Check sheet for the modelled part. Datum: model origin and axes. Units: mm. Coordinates: 2 decimals unless noted, no trailing zeros. Write each loop counter-clockwise with the first axis right and the second up, starting at its lowest first coordinate (ties: lowest second). Pieces come first, ordered by that corner, then holes. Notation, with made-up numbers: (-23.75, 63) -> (-0.75, 63) arc R7 ccw to (-0.75, 73) -> close; hole circle Ø9 at (14, 85.25). An arc over 180 degrees is marked (long way). One line per item, written item: value. Start each with the question number.
1) Draft check along Z on faces 1 (the cylindrical face through (-46.367, 225.4, -60.47)), 2 (the cylindrical face through (23.54, 225.4, 74.74)), 3 (the flat face through (66.1, 0, -38.4)). Enter one of: +Z half, -Z half, draft (parallel to the pull), parting line (faces both ways), or undercut.
2) Sectioned sample at C-C on y = 287.5. Enter the section's corners in (x, z).
3) Sectioned sample at A-A on z = 0. Enter the section's corners in (x, y).
4) Scan lines: line 1 along Z through (x, y) = (0, 292); line 2 along Y through (x, z) = (0, 76.7); line 3 along Z through (x, y) = (52, 426.5). Record each from-to range of solid material in increasing order. Write a range as [from, to].
5) Gauge pin test, flat ends, axial feed: P1, Ø5, axis at x = 19, y = 296, coming from the -Z side; P2, Ø6, axis at x = 62, y = 115, coming from the +Z side; P3, Ø5, axis at x = -47, y = 353.5, coming from the +Z side; P4, Ø2, axis at x = 0, y = 4.76, coming from the -Z side. Record the tip position at first contact, or that the pin passes through.
6) Sectioned sample at B-B on x = 53. Enter the section's corners in (y, z).
```python
from build123d import *

# Parameters (mm, degrees)
SKETCH1_R               = 78.359
SKETCH1_R_2             = 76.2
BOSS_EXTRUDE1_DEPTH     = 457.2
SKETCH2_R               = 1.750000056
CUT_EXTRUDE1_DEPTH      = 471.438206104
CIRPATTERN1_COUNT       = 6
CUT_EXTRUDE2_REACH      = 491.625
CUT_EXTRUDE2_END_RADIUS = 76.2
CIRPATTERN2_COUNT       = 3


with BuildPart() as part:
    # Sketch1 → Boss-Extrude1 (new body)
    with BuildSketch(Plane(origin=(0, 0, 0), x_dir=(1, 0, 0), z_dir=(0, 1, 0))):
        with Locations(Location((0, 0, 0), (0, 0, 270))):
            Circle(SKETCH1_R)
        with Locations(Location((0, 0, 0), (0, 0, 270))):
            Circle(SKETCH1_R_2, mode=Mode.SUBTRACT)
    extrude(amount=BOSS_EXTRUDE1_DEPTH)

    # Sketch2 → Cut-Extrude1 (cut, through all)
    with BuildSketch(Plane.XY):
        with Locations(Location((0, 4.7625, 0), (0, 0, 90))):
            Circle(SKETCH2_R)
    cut_extrude1 = extrude(amount=-CUT_EXTRUDE1_DEPTH, mode=Mode.SUBTRACT)

    # CirPattern1: Cut-Extrude1 ×6 about axis
    cirpattern1_axis = Axis((0, 457.2, 0), (0, -1, 0))
    for i in range(1, CIRPATTERN1_COUNT):
        add(cut_extrude1.rotate(cirpattern1_axis, i * 360 / CIRPATTERN1_COUNT), mode=Mode.SUBTRACT)

    # Cut-Extrude2: up to this cylinder (the profile starts outside it)
    cut_extrude2_end = Plane(origin=(0, 3.909431, 0), z_dir=(0, -1, 0)) * Cylinder(CUT_EXTRUDE2_END_RADIUS, 1136.65, mode=Mode.PRIVATE)
    # Sketch3 → Cut-Extrude2 (cut, up to the surface)
    with BuildSketch(Plane(origin=(0, 0, -78.359), x_dir=(-1, 0, 0), z_dir=(0, 0, -1)), mode=Mode.PRIVATE) as cut_extrude2_sk1:
        with BuildLine():
            Line((-3.81, 4.732887187), (-3.81, 0))
            Line((-3.81, 0), (3.81, 0))
            Line((3.81, 0), (3.81, 4.732887187))
            ThreePointArc((3.81, 4.732887187), (0, 8.542887187), (-3.81, 4.732887187))
        make_face()
    cut_extrude2_tool1 = extrude(cut_extrude2_sk1.sketch, amount=-CUT_EXTRUDE2_REACH, mode=Mode.PRIVATE) - cut_extrude2_end
    cut_extrude2 = cut_extrude2_tool1.solids().sort_by_distance((0, 3.909431, -78.359))[0]
    add(cut_extrude2, mode=Mode.SUBTRACT)

    # CirPattern2: Cut-Extrude2 ×3 about axis
    cirpattern2_axis = Axis((0, 0, 0), (0, 1, 0))
    for i in range(1, CIRPATTERN2_COUNT):
        add(cut_extrude2.rotate(cirpattern2_axis, i * 360 / CIRPATTERN2_COUNT), mode=Mode.SUBTRACT)


solid = part.part
```
Answers:
1. face 1: undercut
1. face 2: parting line
1. face 3: draft
2. outline: circle Ø156.72 at (0, 0); hole circle Ø152.4 at (0, 0)
3. outline: (-78.36, 0) -> (-76.2, 0) -> (-76.2, 457.2) -> (-78.36, 457.2) -> close; (76.2, 0) -> (78.36, 0) -> (78.36, 457.2) -> (76.2, 457.2) -> close
4. line 1: z = [-78.36, -76.2], [76.2, 78.36]
4. line 2: y = [0, 3.01], [6.51, 457.2]
4. line 3: z = [-58.62, -55.7], [55.7, 58.62]
5. P1: stops at z = -76.6
5. P2: stops at z = 51.57
5. P3: stops at z = 64.5
5. P4: passes through
6. outline: (0, -57.72) -> (457.2, -57.72) -> (457.2, -54.75) -> (0, -54.75) -> close; (0, 54.75) -> (457.2, 54.75) -> (457.2, 57.72) -> (0, 57.72) -> close
